```python
from build123d import *

# Parameters (mm, degrees)
SKETCH1_W           = 30
SKETCH1_H           = 74.468085106
BOSS_EXTRUDE1_DEPTH = 25
SKETCH2_R           = 7.415
SKETCH2_R_2         = 3.075
CUT_EXTRUDE1_DEPTH  = 64.7


with BuildPart() as part:
    # Sketch1 → Boss-Extrude1 (new body)
    with BuildSketch(Plane(origin=(0, 0, 0), x_dir=(0, 0, -1), z_dir=(1, 0, 0))):
        Rectangle(SKETCH1_W, SKETCH1_H)
    extrude(amount=BOSS_EXTRUDE1_DEPTH)

    # Sketch2 → Cut-Extrude1 (cut)
    with BuildSketch(Plane(origin=(0, 37.234042553, 0), x_dir=(1, 0, 0), z_dir=(0, 1, 0))):
        with Locations(Location((12.128550828, 0, 0), (0, 0, 270))):
            Circle(SKETCH2_R)
        with Locations(Location((12.128550828, 0, 0), (0, 0, 270))):
            Circle(SKETCH2_R_2, mode=Mode.SUBTRACT)
    extrude(amount=-CUT_EXTRUDE1_DEPTH, mode=Mode.SUBTRACT)


solid = part.part
```
Could you check a few things on this model? Use its own coordinates, in mm. A direction names the side the tool comes from. Coordinates: 2 decimals unless noted, no trailing zeros. Write each loop counter-clockwise with the first axis right and the second up, starting at its lowest first coordinate (ties: lowest second). Pieces come first, ordered by that corner, then holes. Notation, with made-up numbers: (33.25, 86.5) - (65.25, 86.5) arc R24 cw to (65.25, 120.5) - close; hole circle Ø11 at (-22.5, 84.25). An arc over 180 degrees is marked (long way). Use a Markdown table: item, result.
Q1. Imagine slicing it at C-C (x = 18.25). List the corners of the cut face in (y, z) for me.
Geometry check:
| item | result |
|---|---|
| outline | (-37.23, -15) - (37.23, -15) - (37.23, -4.18) - (-27.47, -4.18) - (-27.47, 4.18) - (37.23, 4.18) - (37.23, 15) - (-37.23, 15) - close |
Q2. Imagine slicing it at B-B (y = 4). List the corners of the cut face in (x, z) for me (3 decimals).
Geometry check:
| item | result |
|---|---|
| outline | (0, -15) - (25, -15) - (25, 15) - (0, 15) - close; circle Ø6.15 at (12.129, 0); hole circle Ø14.83 at (12.129, 0) |
Q3. Thinking about a two-plate mould opening in X: for faces 3 (the cylindrical face through (19.48, 5.34, -0.97)), 4 (the flat face through (25, 1, 0)), 5 (the flat face through (15, 37.234, 7)), which applies, +X half, -X half, draft (parallel to the pull), parting line (faces both ways), or undercut?
Geometry check:
| item | result |
|---|---|
| face 3 | undercut |
| face 4 | +X half |
| face 5 | draft |
Q4. Imagine slicing it at A-A (z = 0). List the corners of the cut face in (x, y) for me.
Geometry check:
| item | result |
|---|---|
| outline | (0, -37.23) - (25, -37.23) - (25, 37.23) - (19.54, 37.23) - (19.54, -27.47) - (15.2, -27.47) - (15.2, 37.23) - (9.05, 37.23) - (9.05, -27.47) - (4.71, -27.47) - (4.71, 37.23) - (0, 37.23) - close |
Q5. Please list where these lines run through material, in increasing order: L1, parallel to X at y = 10, z = 0; L2, parallel to X at y = 13, z = -2.75; L3, parallel to Z at x = 9.5, y = -3.5.
Geometry check:
| item | result |
|---|---|
| L1 | x = 0 to 4.71, 9.05 to 15.2, 19.54 to 25 |
| L2 | x = 0 to 5.24, 10.75 to 13.5, 19.01 to 25 |
| L3 | z = -15 to -6.93, -1.6 to 1.6, 6.93 to 15 |
Q6. Which directions (+Z, -Z, +X, -X, +Y, -Y) give clear straight access to the entire face, cutting with the end or side of a thin tool? Please do faces 1 (the flat face through (12, 37.234, 0)), 2 (the flat face through (8.9, -27.466, -0.1)).
Geometry check:
| item | result |
|---|---|
| face 1 | +Z, -Z, +X, -X, +Y |
| face 2 | +Y |
Q7. Imagine slicing it at D-D (z = 6.25). List the corners of the cut face in (x, y) for me.
Geometry check:
| item | result |
|---|---|
| outline | (0, -37.23) - (25, -37.23) - (25, 37.23) - (16.12, 37.23) - (16.12, -27.47) - (8.14, -27.47) - (8.14, 37.23) - (0, 37.23) - close |
